For this review, take the finished solid that the model builds, in its own axes (mm). A direction names the side the tool comes from. Round coordinates to 2 decimals unless told otherwise and drop trailing zeros. Order: outer loops, then holes, each group sorted by start corner. A loop starts at its lowest first (then second) coordinate and runs counter-clockwise, first axis right, second up. Notation, with made-up numbers: M 70,68 L 95,68 A31 ccw 95,97 Z; hole C 25,-24.75 d8. An arc over 180 degrees is marked long. Use a Markdown table: item, result.
from build123d import *

# Parameters (mm, degrees)
SKETCH1_R           = 58.166
BOSS_EXTRUDE1_DEPTH = 21.971
SKETCH3_R           = 51.816
CUT_EXTRUDE2_DEPTH  = 18.796
CUT_EXTRUDE7_DEPTH  = 18.796
SKETCH7_R           = 6.477
BOSS_EXTRUDE3_DEPTH = 10.9855


with BuildPart() as part:
    # Sketch1 → Boss-Extrude1 (new body)
    with BuildSketch(Plane(origin=(0, 0, 0), x_dir=(1, 0, 0), z_dir=(0, 1, 0))):
        Circle(SKETCH1_R)
    extrude(amount=BOSS_EXTRUDE1_DEPTH)

    # Sketch3 → Cut-Extrude2 (cut)
    with BuildSketch(Plane(origin=(0, 21.971, 0), x_dir=(1, 0, 0), z_dir=(0, 1, 0))):
        Circle(SKETCH3_R)
    extrude(amount=-CUT_EXTRUDE2_DEPTH, mode=Mode.SUBTRACT)

    # Sketch6 → Cut-Extrude7 (cut)
    with BuildSketch(Plane(origin=(0, 21.971, 0), x_dir=(1, 0, 0), z_dir=(0, 1, 0))):
        with BuildLine():
            Line((9.363048829, 50.963037318), (9.340756891, 57.411094892))
            ThreePointArc((9.340756891, 57.411094892), (2.903170649, 58.093503563), (-3.57037671, 58.056317194))
            Line((-3.57037671, 58.056317194), (-3.57037671, 51.692845406))
            ThreePointArc((-3.57037671, 51.692845406), (2.919232353, 51.733702153), (9.363048829, 50.963037318))
        make_face()
    extrude(amount=-CUT_EXTRUDE7_DEPTH, mode=Mode.SUBTRACT)

    # Sketch7 → Boss-Extrude3 (add)
    with BuildSketch(Plane.XZ):
        with BuildLine():
            ThreePointArc((55.382885714, -17.776938037), (81.28, 0), (55.382885714, 17.776938037))
            ThreePointArc((55.382885714, 17.776938037), (58.166, 0), (55.382885714, -17.776938037))
        make_face()
        with Locations((68.326, 0)):
            Circle(SKETCH7_R, mode=Mode.SUBTRACT)
        with BuildLine():
            ThreePointArc((-55.382885714, 17.776938037), (-81.28, 0), (-55.382885714, -17.776938037))
            ThreePointArc((-55.382885714, -17.776938037), (-58.166, 0), (-55.382885714, 17.776938037))
        make_face()
        with Locations((-68.323824172, 0)):
            Circle(SKETCH7_R, mode=Mode.SUBTRACT)
    extrude(amount=-BOSS_EXTRUDE3_DEPTH)


solid = part.part
Q1. Add section D-D (y = 6). Write out the cut boundary in (x, z), then the cut area to 3 significant figures.
Determined:
| item | result |
|---|---|
| outline | M -55.38,-17.78 A58.17 ccw -3.57,-58.06 L -3.57,-51.69 A51.82 cw long 9.36,-50.96 L 9.34,-57.41 A58.17 ccw 55.38,-17.78 A19.05 ccw long 55.38,17.78 A58.17 ccw -55.38,17.78 A19.05 ccw long Z; hole C -68.32,0 d12.95; hole C 68.33,0 d12.95 |
| area | 3,370 mm^2 |
Q2. Wall thickness on line 1 along X through (y, z) = (6.5, 5.5); line 2 along X through (y, z) = (18.5, 4); line 3 along Z through (x, y) = (-71.5, 4.5): over which ranges is each line inside the solid? List them lowest first. Write a range as [from, to].
Determined:
| item | result |
|---|---|
| line 1 | x = [-80.47, -71.74], [-64.9, -51.52], [51.52, 64.91], [71.75, 80.47] |
| line 2 | x = [-58.03, -51.66], [51.66, 58.03] |
| line 3 | z = [-16.64, -5.64], [5.64, 16.64] |
Q3. Add section B-B (x = 0). Write out the cut boundary in (y, z) (3 decimals).
Determined:
| item | result |
|---|---|
| outline | M 0,-58.166 L 3.175,-58.166 L 3.175,51.816 L 21.971,51.816 L 21.971,58.166 L 0,58.166 Z |
Q4. Clearance check with flat-ended pins moving along their axes: pin 1 (7 mm diameter, centred on y = 15.5, z = -54, fed in from +X); pin 2 (1 mm diameter, centred on y = 4.5, z = -38, fed in from -X); pin 3 (3 mm diameter, centred on y = 15.5, z = -14.5, fed in from +X). State where each tip first meets the part, or that it passes through.
Determined:
| item | result |
|---|---|
| pin 1 | stops at x = 28.86 |
| pin 2 | stops at x = -44.46 |
| pin 3 | stops at x = 56.69 |
Q5. Draft analysis for pull direction Z (two halves, no side actions). For faces 4 (the flat face through (-1, 3.175, -4)), 5 (the cylindrical face through (26.84, 10.832, 51.603)), 6 (the flat face through (-63, 10.986, -4)), state which applies: pulls with the +Z half, pulls with the -Z half, needs draft (parallel to the pull), parting line crosses it, or undercut.
Determined:
| item | result |
|---|---|
| face 4 | undercut |
| face 5 | parting line crosses it |
| face 6 | needs draft |
Q6. Add section C-C (x = -68). Write out the cut boundary in (y, z), then the cut area to 3 significant figures.
Determined:
| item | result |
|---|---|
| outline | M 0,-18.16 L 10.99,-18.16 L 10.99,-6.47 L 0,-6.47 Z; M 0,6.47 L 10.99,6.47 L 10.99,18.16 L 0,18.16 Z |
| area | 257 mm^2 |
Q7. Machinability: for faces 1 (the flat face through (-35, 21.971, 39)), 2 (the cylindrical face through (-5.101, 12.705, 51.564)), 3 (the flat face through (-3.57, 13, -55)), which of the approach directions +Z, -Z, +X, -X, +Y, -Y give a long, thin tool a straight path to every point of the face, cutting with its end or side? Answer none if there is none.
Determined:
| item | result |
|---|---|
| face 1 | +Z, -Z, +X, -X, +Y |
| face 2 | +Y |
| face 3 | -Z, +Y |
Q8. Add section A-A (z = 0). Write out the cut boundary in (x, y) (1 decimal).
Determined:
| item | result |
|---|---|
| outline | M -81.3,0 L -74.8,0 L -74.8,11 L -81.3,11 Z; M -61.8,0 L 61.8,0 L 61.8,11 L 58.2,11 L 58.2,22 L 51.8,22 L 51.8,3.2 L -51.8,3.2 L -51.8,22 L -58.2,22 L -58.2,11 L -61.8,11 Z; M 74.8,0 L 81.3,0 L 81.3,11 L 74.8,11 Z |
